```python
from build123d import *

# Parameters (mm, degrees)
SKETCH_1_W      = 9
SKETCH_1_H      = 9
EXTRUDE_1_DEPTH = 5.4
SKETCH_2_W      = 2.9
SKETCH_2_H      = 3
EXTRUDE_2_DEPTH = 3.9
EXTRUDE_3_DEPTH = 2


with BuildPart() as part:
    # 스케치1 → 보스-돌출1 (new body)
    with BuildSketch(Plane.XY):
        with Locations((4.5, 4.5)):
            Rectangle(SKETCH_1_W, SKETCH_1_H)
    extrude(amount=EXTRUDE_1_DEPTH)

    # 스케치2 → 보스-돌출2 (add)
    with BuildSketch(Plane(origin=(0, 0, 0), x_dir=(-1, 0, 0), z_dir=(0, 0, -1))):
        with Locations((1.45, 4.5)):
            Rectangle(SKETCH_2_W, SKETCH_2_H)
        with Locations((-10.45, 4.5)):
            Rectangle(SKETCH_2_W, SKETCH_2_H)
    extrude(amount=-EXTRUDE_2_DEPTH)

    # 스케치3 → 보스-돌출3 (add, symmetric)
    with BuildSketch(Plane(origin=(0, 4.5, 0), x_dir=(1, 0, 0), z_dir=(0, 1, 0))):
        with BuildLine():
            Line((3.577763231, 4), (3.577763231, 5))
            Line((3.577763231, 5), (5.422236769, 5))
            Line((5.422236769, 5), (5.422236769, 4))
            ThreePointArc((5.422236769, 4), (4.794518093, 2), (5.422236769, 0))
            Line((5.422236769, 0), (3.577763231, 0))
            ThreePointArc((3.577763231, 0), (4.205481907, 2), (3.577763231, 4))
        make_face()
    extrude(amount=EXTRUDE_3_DEPTH, both=True)


solid = part.part
```
Build history of the part. All positions in model axes, mm. A direction names the side the tool comes from. Round coordinates to 2 decimals unless told otherwise and drop trailing zeros. Order: outer loops, then holes, each group sorted by start corner. A loop starts at its lowest first (then second) coordinate and runs counter-clockwise, first axis right, second up. Notation, with made-up numbers: (-22, 37.5) -> (14, 37.5) arc R27 cw to (14, 59.5) -> close; hole circle Ø3 at (66, 22). An arc over 180 degrees is marked (long way). Answer in a Markdown table with one row per item.
1) Which spindle directions (+Z, -Z, +X, -X, +Y, -Y) get a long thin tool onto all of the face, cutting with end or side? Do faces 4 (the flat face through (4.5, 6.5, -3.1)), 5 (the flat face through (10, 3, 2)), 6 (the flat face through (10, 5, 3.9)), 7 (the flat face through (10, 6, 2)). Say none if no direction does.
Values:
| item | result |
|---|---|
| face 4 | -Z, +X, -X, +Y |
| face 5 | +Z, -Z, +X, -Y |
| face 6 | +Z, +X, +Y, -Y |
| face 7 | +Z, -Z, +X, +Y |
2) Band-saw the part on A-A on z = 3. Give the cut face in (x, y).
Values:
| item | result |
|---|---|
| outline | (-2.9, 3) -> (0, 3) -> (0, 0) -> (9, 0) -> (9, 3) -> (11.9, 3) -> (11.9, 6) -> (9, 6) -> (9, 9) -> (0, 9) -> (0, 6) -> (-2.9, 6) -> close |
3) Wall check: L1, parallel to Z at x = 6, y = 7.75; L2, parallel to X at y = 0.5, z = 4.25; L3, parallel to Y at x = 9.5, z = 2. Give the ranges that are in metal, low to high.
Values:
| item | result |
|---|---|
| L1 | 0 to 5.4 |
| L2 | 0 to 9 |
| L3 | 3 to 6 |
4) Band-saw the part on B-B on y = 4.75. Give the cut face in (x, z), and give its area (3 significant figures).
Values:
| item | result |
|---|---|
| outline | (-2.9, 0) -> (3.58, 0) arc R3.5 cw to (3.58, -4) -> (3.58, -5) -> (5.42, -5) -> (5.42, -4) arc R3.5 cw to (5.42, 0) -> (11.9, 0) -> (11.9, 3.9) -> (9, 3.9) -> (9, 5.4) -> (0, 5.4) -> (0, 3.9) -> (-2.9, 3.9) -> close |
| area | 77.0 mm2 |
5) Band-saw the part on C-C on x = 7.5. Give the cut face in (y, z), and give its area (3 significant figures).
Values:
| item | result |
|---|---|
| outline | (0, 0) -> (9, 0) -> (9, 5.4) -> (0, 5.4) -> close |
| area | 48.6 mm2 |
6) Pin check, flat tips, straight feed: P1, Ø0.9, axis at x = 11, y = 4.5, coming from the +Z side; P2, Ø2.5, axis at x = -2, z = 1, coming from the -Y side; P3, Ø2.5, axis at x = 10.5, z = 1.5, coming from the +Y side; P4, Ø2, axis at x = 8, z = 1, coming from the -Y side. Stop position of each tip, or through.
Values:
| item | result |
|---|---|
| P1 | z = 3.9 |
| P2 | y = 3 |
| P3 | y = 6 |
| P4 | y = 0 |
7) Mould opens along Z. For faces 1 (the flat face through (-1, 5, 3.9)), 2 (the cylindrical face through (4.795, 4.528, -2.03)), 3 (the flat face through (5.422, 4.5, -4.5)) say: released by +Z, released by -Z, zero draft, split by the parting line, or undercut.
Values:
| item | result |
|---|---|
| face 1 | released by +Z |
| face 2 | undercut |
| face 3 | zero draft |
